from build123d import *

# Parameters (mm, degrees)
SKETCH3_R          = 35.304496673
CUT_EXTRUDE2_DEPTH = 25
CUT_EXTRUDE2_DRAFT = -37


with BuildPart() as part:
    # Sketch1 → Revolve1 (revolve)
    with BuildSketch(Plane.XY, mode=Mode.PRIVATE) as revolve1_sk:
        Polygon((0, 0), (-23.668379582, 0), (-27.829852915, 4.161473333), (-72.305599163, 4.161473333), (-75.946888329, 7.8027625), (0, 7.8027625), align=None)
    revolve(revolve1_sk.sketch.rotate(Axis((0, 0, 0), (0, 1, 0)), 270), axis=Axis((0, 0, 0), (0, 1, 0)))

    # Sketch2 → Revolve2 (revolve)
    with BuildSketch(Plane.XY, mode=Mode.PRIVATE) as revolve2_sk:
        with BuildLine():
            Line((-41.476502692, 32.102501356), (0, 32.102501356))
            Line((0, 32.102501356), (0, 7.8027625))
            Line((0, 7.8027625), (-38.491451362, 7.8027625))
            ThreePointArc((-38.491451362, 7.8027625), (-29.235303405, 21.273030582), (-41.476502692, 32.102501356))
        make_face()
    revolve(revolve2_sk.sketch.rotate(Axis((0, 0, 0), (0, 1, 0)), 270), axis=Axis((0, 0, 0), (0, 1, 0)))


with BuildPart() as cut_extrude2_tool:
    # Sketch3 → Cut-Extrude2 (with draft: the straight prism first)
    with BuildSketch(Plane(origin=(0, 32.102501356, 0), x_dir=(1, 0, 0), z_dir=(0, 1, 0))):
        Circle(SKETCH3_R)
    extrude(amount=-CUT_EXTRUDE2_DEPTH)
    # Cut-Extrude2: the draft: its side faces are tilted about the plane it starts from
    cut_extrude2_sides = [cut_extrude2_tool.faces().sort_by_distance(p)[0] for p in [
        (-35.304496673, 19.602501356, 0),
    ]]
    draft(cut_extrude2_sides, Plane(origin=(0, 32.102501356, 0), x_dir=(1, 0, 0), z_dir=(0, 1, 0)), CUT_EXTRUDE2_DRAFT)


with BuildPart() as part_1:
    add(part.part)

    # Cut-Extrude2: cut by cut_extrude2_tool
    add(cut_extrude2_tool.part, mode=Mode.SUBTRACT)


solid = part_1.part
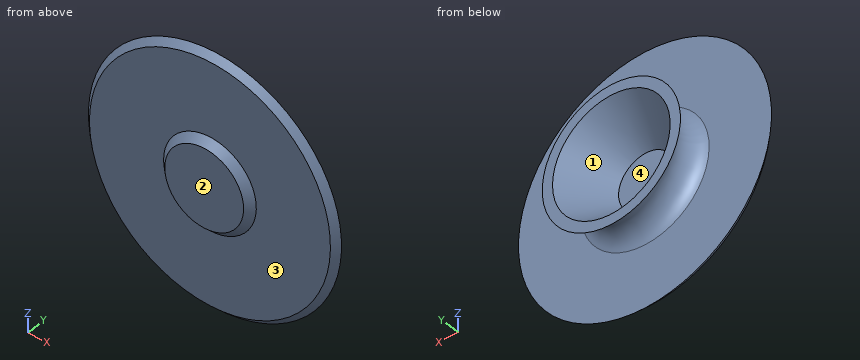
Build history of the part. All positions in model axes, mm. Face numbers are marked on the shaded views. A direction names the side the tool comes from. Coordinates: 2 decimals unless noted, no trailing zeros. Order: outer loops, then holes, each group sorted by start corner. A loop starts at its lowest first (then second) coordinate and runs counter-clockwise, first axis right, second up. Notation, with made-up numbers: (75, 34.5) - (100, 34.5) arc R9 ccw to (100, 48.5) - close; hole circle Ø11 at (52.5, -18.5). An arc over 180 degrees is marked (long way). Write each question's results on one line, items separated by ' | '. Start each with the question number.
Item 1: Tool access for the marked faces 3 and 4: list every direction of +Z, -Z, +X, -X, +Y, -Y with a clear straight run to the whole face (end or side of a thin tool).
Item 2: Band-saw the part on C-C on y = 19.5. Write the cut outline in (x, z).
Item 3: Flat gauge pins, fed straight in: pin 1 (12 mm diameter, centred on x = 50, z = 46.5, fed in from +Y); pin 2 (3 mm diameter, centred on x = 10, y = 14.5, fed in from +Z). Where does each tip first touch, or does it go through?
Item 4: Band-saw the part on D-D on y = 11. Write the cut outline in (x, z), and give its area (3 significant figures).
Item 5: Wall check: probe 1 along Y at (x, z) = (-40, -51.5); probe 2 along Z at (x, y) = (12, 17); probe 3 along X at (y, z) = (17.5, -21). Give the ranges that are in metal, low to high. Write a range as [from, to].
Item 6: Band-saw the part on B-B on z = 0. Write the cut outline in (x, y).
Item 7: Mould opens along X. For the marked faces 1 and 2 say: released by +X, released by -X, zero draft, split by the parting line, or undercut.
Item 8: Band-saw the part on A-A on x = 0. Write the cut outline in (y, z).
Numbers:
1) face 3: -Y | face 4: +Y
2) outline: circle Ø58.29 at (0, 0); hole circle Ø51.62 at (0, 0)
3) pin 1: y = 7.8 | pin 2: z = 29.63
4) outline: circle Ø65.61 at (0, 0); hole circle Ø38.81 at (0, 0) | area: 2,200 mm^2
5) probe 1: [4.16, 7.8] | probe 2: [-26.9, -20.7], [20.7, 26.9] | probe 3: [-20.51, -12.23], [12.23, 20.51]
6) outline: (-75.95, 7.8) - (-72.31, 4.16) - (-27.83, 4.16) - (-23.67, 0) - (23.67, 0) - (27.83, 4.16) - (72.31, 4.16) - (75.95, 7.8) - (38.49, 7.8) arc R12.33 cw to (41.48, 32.1) - (35.3, 32.1) - (16.47, 7.1) - (-16.47, 7.1) - (-35.3, 32.1) - (-41.48, 32.1) arc R12.33 cw to (-38.49, 7.8) - close
7) face 1: undercut | face 2: zero draft
8) outline: (0, -23.67) - (4.16, -27.83) - (4.16, -72.31) - (7.8, -75.95) - (7.8, -38.49) arc R12.33 cw to (32.1, -41.48) - (32.1, -35.3) - (7.1, -16.47) - (7.1, 16.47) - (32.1, 35.3) - (32.1, 41.48) arc R12.33 cw to (7.8, 38.49) - (7.8, 75.95) - (4.16, 72.31) - (4.16, 27.83) - (0, 23.67) - close
